```python
from build123d import *

# Parameters (mm, degrees)
F1_DEPTH = 95.25
F2_R     = 9.52499
F3_R     = 3.175
F4_DEPTH = 95.251


# Not quite as in the source:
# - a fillet or chamfer is up to 0.001 mm smaller than in the source, because OpenCascade refuses the exact size
# - a feature names something its author has since deleted; it is built from what else it names


with BuildPart() as f1:
    # F0 (on Front) → F1 (new body)
    with BuildSketch(Plane.XZ):
        Polygon((-12.472799319, 39.8380596402), (-31.522799319, 39.8380596402), (-31.522799319, -30.0119403598), (7.847200681, -30.0119403598), (7.847200681, -10.9619403598), (-12.472799319, -10.9619403598), align=None)
    extrude(amount=F1_DEPTH)

    # F2 (radius 9.525 in the source; OpenCascade refuses exactly that, so slightly less here)
    f2_edges = [f1.edges().sort_by_distance(p)[0] for p in [
        (7.847201, -47.625, -10.96194),
        (7.847201, -47.625, -30.01194),
    ]]
    fillet(f2_edges, radius=F2_R)

    # F3 (on face) → F4 (cut, through all)
    with BuildSketch(Plane.XZ.offset(95.25)):
        with Locations((-1.677799319, -20.4869403598)):
            Circle(F3_R)
    extrude(amount=-F4_DEPTH, mode=Mode.SUBTRACT)


solid = f1.part
```
Input: part model. Units: mm. Frame: model coordinates. Give positions to 0.01 mm unless a question says otherwise; leave off trailing zeros. Order: outer loops, then holes, each group sorted by start corner. A loop starts at its lowest first (then second) coordinate and runs counter-clockwise, first axis right, second up. Notation, with made-up numbers: M 23.25,87.5 L 70.25,87.5 A19 cw 70.25,91.5 Z; hole C 15.5,69 d7. An arc over 180 degrees is marked long. One line per question, with ' | ' between items. Start each with the question number.
1. First-contact query: pin 1 Ø8.5 at (x, y) = (-6.5, -35) entering from +Z; pin 2 Ø8 at (y, z) = (-31.5, 12.5) entering from +X. Flat tips, straight axial feed; report the tip coordinate or a pass-through.
2. Section query D-D (z = 16). Return the cut outline in (x, y).
3. Material intervals for probe 1 along Z at (x, y) = (-1.5, -87.5); probe 2 along Z at (x, y) = (-8, -17.5); probe 3 along X at (y, z) = (-19, 33), sorted ascending. Write a range as [from, to].
4. Section query C-C (x = -8). Return the cut outline in (y, z).
5. Section query B-B (z = -19). Return the cut outline in (x, y).
6. Pull-direction query (X, two-part tool) for faces 1 (the face through (-7, -47, -10.962)), 2 (the face through (-2.09, -48.29, -17.34)), 3 (the face through (-12.473, -47, 14)); classes: released by +X, released by -X, zero draft, split by the parting line, or undercut.
Here are the results:
1) pin 1: z = -10.96 | pin 2: x = -12.47
2) outline: M -31.52,-95.25 L -12.47,-95.25 L -12.47,0 L -31.52,0 Z
3) probe 1: [-30.01, -23.66], [-17.32, -10.96] | probe 2: [-30.01, -10.96] | probe 3: [-31.52, -12.47]
4) outline: M -95.25,-30.01 L 0,-30.01 L 0,-10.96 L -95.25,-10.96 Z
5) outline: M -31.52,-95.25 L -4.48,-95.25 L -4.48,0 L -31.52,0 Z; M 1.13,-95.25 L 7.73,-95.25 L 7.73,0 L 1.13,0 Z
6) face 1: zero draft | face 2: undercut | face 3: released by +X
